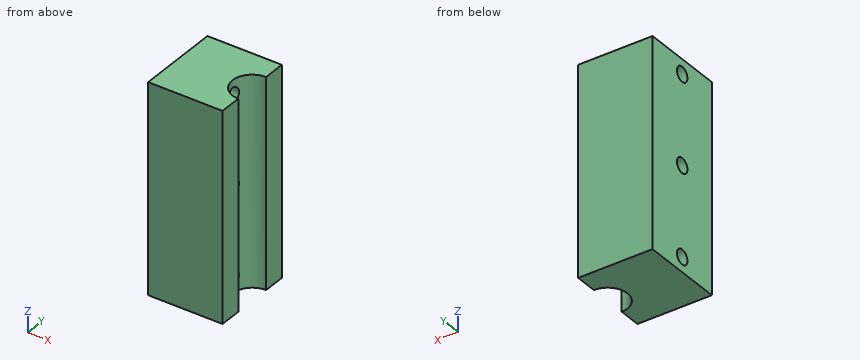
```python
from build123d import *

# Parameters (mm, degrees)
BOSS_EXTRUDE1_DEPTH = 70
SKETCH2_R           = 2.5
CUT_EXTRUDE1_DEPTH  = 76.660528844


with BuildPart() as part:
    # Sketch1 → Boss-Extrude1 (new body)
    with BuildSketch(Plane.XY):
        with BuildLine():
            Line((0, 6.625), (0, 14.125))
            Line((0, 14.125), (-25, 14.125))
            Line((-25, 14.125), (-25, -14.125))
            Line((-25, -14.125), (0, -14.125))
            Line((0, -14.125), (0, -6.625))
            ThreePointArc((0, -6.625), (-6.625, 0), (0, 6.625))
        make_face()
    extrude(amount=BOSS_EXTRUDE1_DEPTH)

    # Sketch2 → Cut-Extrude1 (cut, through all)
    with BuildSketch(Plane.ZY.offset(25)):
        with Locations((5, 0)):
            Circle(SKETCH2_R)
        with Locations((35, 0)):
            Circle(SKETCH2_R)
        with Locations((65, 0)):
            Circle(SKETCH2_R)
    extrude(amount=-CUT_EXTRUDE1_DEPTH, mode=Mode.SUBTRACT)


solid = part.part
```
Input: part model. Units: mm. Frame: model coordinates. Coordinates: 2 decimals unless noted, no trailing zeros. Write each loop counter-clockwise with the first axis right and the second up, starting at its lowest first coordinate (ties: lowest second). Pieces come first, ordered by that corner, then holes. Notation, with made-up numbers: (7, -37) -> (24, -37) arc R35 cw to (24, -4) -> close; hole circle Ø5 at (-17, 47). An arc over 180 degrees is marked (long way). Answer as a JSON object with one key per item and string values.
1. First-contact query: P1, Ø4.5, axis at y = 0, z = 65, coming from the -X side; P2, Ø8, axis at y = 0, z = 35, coming from the +X side. Flat tips, straight axial feed; report the tip coordinate or a pass-through.
Result set:
{"P1": "passes through", "P2": "stops at x = -5.28"}
2. Section D-D on x = -3.25. Return the cut outline in (y, z) (3 decimals), then the cut area to 3 significant figures.
Result set:
{"outline": "(-14.125, 0) -> (-5.773, 0) -> (-5.773, 70) -> (-14.125, 70) -> close; (5.773, 0) -> (14.125, 0) -> (14.125, 70) -> (5.773, 70) -> close", "area": "1,170 mm2"}
3. Section C-C on y = 0. Return the cut outline in (x, z) (3 decimals).
Result set:
{"outline": "(-25, 0) -> (-6.625, 0) -> (-6.625, 2.5) -> (-25, 2.5) -> close; (-25, 7.5) -> (-6.625, 7.5) -> (-6.625, 32.5) -> (-25, 32.5) -> close; (-25, 37.5) -> (-6.625, 37.5) -> (-6.625, 62.5) -> (-25, 62.5) -> close; (-25, 67.5) -> (-6.625, 67.5) -> (-6.625, 70) -> (-25, 70) -> close"}
4. Section B-B on x = -15.5. Return the cut outline in (y, z) (3 decimals).
Result set:
{"outline": "(-14.125, 0) -> (14.125, 0) -> (14.125, 70) -> (-14.125, 70) -> close; hole circle Ø5 at (0, 5); hole circle Ø5 at (0, 35); hole circle Ø5 at (0, 65)"}
5. Material intervals for line 1 (Z direction, x = -14.5, y = 0); line 2 (Y direction, x = -21, z = 65) (3 decimals); line 3 (X direction, y = -4.5, z = 34.5), sorted ascending. Write a range as from..to.
Result set:
{"line 1": "z = 0..2.5, 7.5..32.5, 37.5..62.5, 67.5..70", "line 2": "y = -14.125..-2.5, 2.5..14.125", "line 3": "x = -25..-4.86"}
6. Section A-A on z = 65. Return the cut outline in (x, y) (3 decimals), then the cut area to 3 significant figures.
Result set:
{"outline": "(-25, -14.125) -> (0, -14.125) -> (0, -6.625) arc R6.625 cw to (-6.135, -2.5) -> (-25, -2.5) -> close; (-25, 2.5) -> (-6.135, 2.5) arc R6.625 cw to (0, 6.625) -> (0, 14.125) -> (-25, 14.125) -> close", "area": "545 mm2"}
